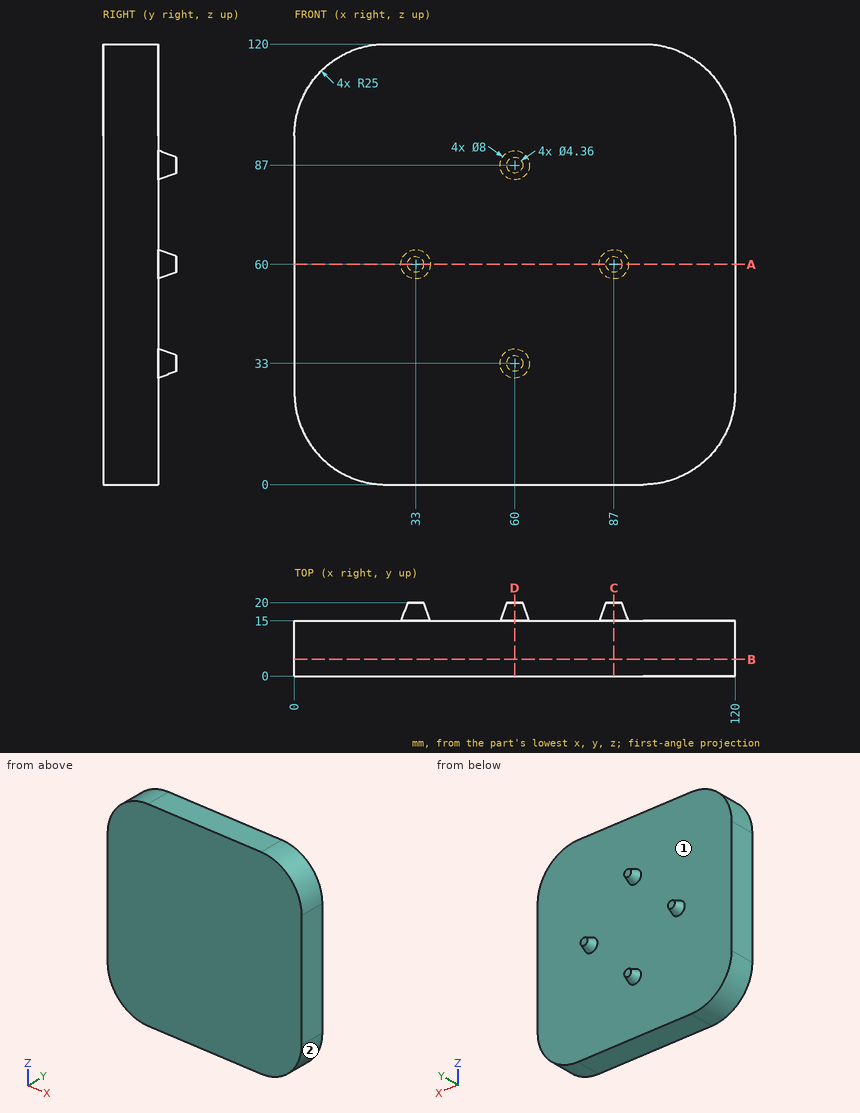
Check sheet for the drawn part. Datum: minimum x, y, z corner. Units: mm. A direction names the side the tool comes from. Round coordinates to 2 decimals unless told otherwise and drop trailing zeros. Write each loop counter-clockwise with the first axis right and the second up, starting at its lowest first coordinate (ties: lowest second). Pieces come first, ordered by that corner, then holes. Notation, with made-up numbers: (-27.75, -7) - (-3.75, -7) arc R21 ccw to (-3.75, 10) - close; hole circle Ø3 at (54, -36). An arc over 180 degrees is marked (long way). Return JSON: item names as keys, results as strings.
Q1. Cross-section at A-A (z = 60). Record the boundary of the cut face in (x, y).
Returned:
{"outline": "(0, 0) - (120, 0) - (120, 15) - (91, 15) - (89.18, 20) - (84.82, 20) - (83, 15) - (37, 15) - (35.18, 20) - (30.82, 20) - (29, 15) - (0, 15) - close"}
Q2. Depth check by flat-ended pin: P1, Ø12, axis at x = 19.5, y = 17, coming from the +Z side; P2, Ø5, axis at y = 11.5, z = 106.5, coming from the -X side; P3, Ø2, axis at y = 14.5, z = 101, coming from the -X side (1 decimal). Enter the tip coordinate at first touch or a pass-through.
Returned:
{"P1": "stops at z = 120", "P2": "stops at x = 1.68", "P3": "stops at x = 0.5"}
Q3. Access from +Z, -Z, +X, -X, +Y, -Y to the whole of each face (thin tool, end or side, straight path). Record for the marked faces 1 and 2.
Returned:
{"face 1": "+Y", "face 2": "-Z, +X, +Y, -Y"}
Q4. Cross-section at B-B (y = 4.5). Record the boundary of the cut face in (x, z).
Returned:
{"outline": "(0, 25) arc R25 ccw to (25, 0) - (95, 0) arc R25 ccw to (120, 25) - (120, 95) arc R25 ccw to (95, 120) - (25, 120) arc R25 ccw to (0, 95) - close"}
Q5. Scan lines: L1, parallel to Y at x = 62.5, z = 26; L2, parallel to X at y = 7.25, z = 96; L3, parallel to Z at x = 9, y = 7.75. Record each from-to range of solid material in increasing order. Write a range as from..to.
Returned:
{"L1": "y = 0..15", "L2": "x = 0.02..119.98", "L3": "z = 5.79..114.21"}
Q6. Cross-section at D-D (x = 60). Record the boundary of the cut face in (y, z).
Returned:
{"outline": "(0, 0) - (15, 0) - (15, 29) - (20, 30.82) - (20, 35.18) - (15, 37) - (15, 83) - (20, 84.82) - (20, 89.18) - (15, 91) - (15, 120) - (0, 120) - close"}
Q7. Cross-section at C-C (x = 87). Record the boundary of the cut face in (y, z).
Returned:
{"outline": "(0, 0) - (15, 0) - (15, 56) - (20, 57.82) - (20, 62.18) - (15, 64) - (15, 120) - (0, 120) - close"}
